from build123d import *

# Parameters (mm, degrees)
SKETCH1_W                     = 300
SKETCH1_H                     = 80
BOSS_EXTRUDE1_DEPTH           = 9.525
SKETCH5_R                     = 8
CUT_EXTRUDE1_DEPTH            = 156.533680034
FILLET1_SIZE                  = 15
M5X0_8_START                  = -1
M5X0_8_TAPPED_HOLE1_OUTLINE_R = 2.1
M5X0_8_TAPPED_HOLE1_DEPTH     = 12
M6_CLEARANCE_HOLE1_D          = 6.4


with BuildPart() as part:
    # Sketch1 → Boss-Extrude1 (new body)
    with BuildSketch(Plane(origin=(0, 0, 0), x_dir=(1, 0, 0), z_dir=(0, 1, 0))):
        Rectangle(SKETCH1_W, SKETCH1_H)
    extrude(amount=BOSS_EXTRUDE1_DEPTH)

    # Sketch5 → Cut-Extrude1 (cut, through all)
    with BuildSketch(Plane(origin=(0, 9.525, 0), x_dir=(1, 0, 0), z_dir=(0, 1, 0))):
        with Locations(Location((-72, 0, 0), (0, 0, 270))):
            Circle(SKETCH5_R)
        with Locations(Location((72, 0, 0), (0, 0, 270))):
            Circle(SKETCH5_R)
    extrude(amount=-CUT_EXTRUDE1_DEPTH, mode=Mode.SUBTRACT)

    # Fillet1
    # a fillet whose section is not a circle: 15 mm, written as the material it takes off along each edge
    with BuildSketch(Plane(origin=(150, -37.5, 40), x_dir=(0, 0, -1), z_dir=(0, 1, 0)), Plane(origin=(150, -37.5, -40), x_dir=(-1, 0, 0), z_dir=(0, 1, 0))) as fillet1_piece_1:
        with BuildLine():
            add(Edge.make_bspline([(FILLET1_SIZE, 0), (FILLET1_SIZE * 0.831801948466, 0), (FILLET1_SIZE * 0.663603896932, 0), (FILLET1_SIZE * 0.292893218813, FILLET1_SIZE * 0.0716919198361), (FILLET1_SIZE * 0.0716919198361, FILLET1_SIZE * 0.292893218813), (0, FILLET1_SIZE * 0.663603896932), (0, FILLET1_SIZE * 0.831801948466), (0, FILLET1_SIZE)], knots=[0, 0, 0, 0, 0, 0, 0.5, 0.5, 1, 1, 1, 1, 1, 1], degree=5))
            Line((0, FILLET1_SIZE), (0, 0))
            Line((0, 0), (FILLET1_SIZE, 0))
        make_face()
    extrude(amount=84.525, mode=Mode.SUBTRACT)
    with BuildSketch(Plane(origin=(-150, -37.5, -40), x_dir=(1, 0, 0), z_dir=(0, 1, 0)), Plane(origin=(-150, -37.5, 40), x_dir=(0, 0, -1), z_dir=(0, 1, 0))) as fillet1_piece_2:
        with BuildLine():
            add(Edge.make_bspline([(FILLET1_SIZE, 0), (FILLET1_SIZE * 0.831801948466, 0), (FILLET1_SIZE * 0.663603896932, 0), (FILLET1_SIZE * 0.292893218813, -FILLET1_SIZE * 0.0716919198361), (FILLET1_SIZE * 0.0716919198361, -FILLET1_SIZE * 0.292893218813), (0, -FILLET1_SIZE * 0.663603896932), (0, -FILLET1_SIZE * 0.831801948466), (0, -FILLET1_SIZE)], knots=[0, 0, 0, 0, 0, 0, 0.5, 0.5, 1, 1, 1, 1, 1, 1], degree=5))
            Line((0, -FILLET1_SIZE), (0, 0))
            Line((0, 0), (FILLET1_SIZE, 0))
        make_face()
    extrude(amount=84.525, mode=Mode.SUBTRACT)

    # M5x0.8 Tapped Hole1: read off the stored shape, not the designer's step
    # M5x0.8 Tapped Hole1 outline → M5x0.8 Tapped Hole1 (cut)
    with BuildSketch(Plane(origin=(0, 0, 0), x_dir=(1, 0, 0), z_dir=(0, 1, 0)).offset(M5X0_8_START)):
        with Locations((57, 23)):
            Circle(M5X0_8_TAPPED_HOLE1_OUTLINE_R)
        with Locations((72, -23)):
            Circle(M5X0_8_TAPPED_HOLE1_OUTLINE_R)
        with Locations((57, -23)):
            Circle(M5X0_8_TAPPED_HOLE1_OUTLINE_R)
        with Locations((72, 23)):
            Circle(M5X0_8_TAPPED_HOLE1_OUTLINE_R)
        with Locations((-57, -23)):
            Circle(M5X0_8_TAPPED_HOLE1_OUTLINE_R)
        with Locations((-72, 23)):
            Circle(M5X0_8_TAPPED_HOLE1_OUTLINE_R)
        with Locations((-57, 23)):
            Circle(M5X0_8_TAPPED_HOLE1_OUTLINE_R)
        with Locations((-72, -23)):
            Circle(M5X0_8_TAPPED_HOLE1_OUTLINE_R)
    extrude(amount=M5X0_8_TAPPED_HOLE1_DEPTH, mode=Mode.SUBTRACT)

    # M6 Clearance Hole1 (through all)
    with Locations(Plane(origin=(0, 0, 0), x_dir=(-1, 0, 0), z_dir=(0, -1, 0))):
        with Locations((132.5, -12.5), (107.5, -12.5), (132.5, 12.5), (107.5, 12.5), (-107.5, -12.5), (-107.5, 12.5), (-132.5, -12.5), (-132.5, 12.5), (34.5, -12.5), (34.5, 12.5), (-34.5, -12.5), (-34.5, 12.5)):
            Hole(M6_CLEARANCE_HOLE1_D / 2)


solid = part.part
The listing builds one solid part. Answer for the finished solid, in the listing's coordinates (mm). Give positions to 0.01 mm unless a question says otherwise; leave off trailing zeros. Order: outer loops, then holes, each group sorted by start corner. A loop starts at its lowest first (then second) coordinate and runs counter-clockwise, first axis right, second up. Notation, with made-up numbers: (-5.5, -7) - (19.5, -7) arc R38 ccw to (19.5, 32) - close; hole circle Ø2 at (34.25, -38). An arc over 180 degrees is marked (long way). Use one line per item in the form item = value.
1) Find section B-B on x = -132.5. Determine the outline of the cut face in (y, z) (3 decimals).
Verdict:
outline = (0, -40) - (9.525, -40) - (9.525, -15.7) - (0, -15.7) - close; (0, -9.3) - (9.525, -9.3) - (9.525, 9.3) - (0, 9.3) - close; (0, 15.7) - (9.525, 15.7) - (9.525, 40) - (0, 40) - close
2) Find section D-D on y = 3.5. Give the number of separate pieces and of enclosed holes in the cut face, and give its area (3 significant figures).
Verdict:
separate_pieces = 1
enclosed_holes = 22
area = 23,000 mm^2
3) The mould has two halves that part along X. Classify faces 1 (the flat face through (-2, 9.525, -1)), 2 (the flat face through (-150, 5, 0)), 3 (the cylindrical face through (135.552, 4.829, -13.461)): released by +X, released by -X, zero draft, split by the parting line, or undercut.
Verdict:
face_1 = zero draft
face_2 = released by -X
face_3 = undercut
4) Find section A-A on z = 0. Determine the outline of the cut face in (x, y) (3 decimals).
Verdict:
outline = (-150, 0) - (-80, 0) - (-80, 9.525) - (-150, 9.525) - close; (-64, 0) - (64, 0) - (64, 9.525) - (-64, 9.525) - close; (80, 0) - (150, 0) - (150, 9.525) - (80, 9.525) - close
5) Consider probe 1 along Z at (x, y) = (132.5, 6.25); probe 2 along X at (y, z) = (7, 0); probe 3 along X at (y, z) = (9.25, -24). Determine where each line is inside the solid, lowest interval first. Write a range as [from, to].
Verdict:
probe_1 = [-40, -15.7], [-9.3, 9.3], [15.7, 40]
probe_2 = [-150, -80], [-64, 64], [80, 150]
probe_3 = [-150, -73.85], [-70.15, -58.85], [-55.15, 55.15], [58.85, 70.15], [73.85, 150]
6) Find section C-C on z = -12.5. Determine the outline of the cut face in (x, y) (3 decimals), and give its area (3 significant figures).
Verdict:
outline = (-150, 0) - (-135.7, 0) - (-135.7, 9.525) - (-150, 9.525) - close; (-129.3, 0) - (-110.7, 0) - (-110.7, 9.525) - (-129.3, 9.525) - close; (-104.3, 0) - (-37.7, 0) - (-37.7, 9.525) - (-104.3, 9.525) - close; (-31.3, 0) - (31.3, 0) - (31.3, 9.525) - (-31.3, 9.525) - close; (37.7, 0) - (104.3, 0) - (104.3, 9.525) - (37.7, 9.525) - close; (110.7, 0) - (129.3, 0) - (129.3, 9.525) - (110.7, 9.525) - close; (135.7, 0) - (150, 0) - (150, 9.525) - (135.7, 9.525) - close
area = 2,490 mm^2
